Could you check a few things on this model? Use its own coordinates, in mm. A direction names the side the tool comes from. Coordinates: 2 decimals unless noted, no trailing zeros. Write each loop counter-clockwise with the first axis right and the second up, starting at its lowest first coordinate (ties: lowest second). Pieces come first, ordered by that corner, then holes.
```python
from build123d import *

# Parameters (mm, degrees)
BOSS_EXTRUDE1_DEPTH = 45.45
CUT_EXTRUDE4_DEPTH  = 1
CUT_EXTRUDE5_DEPTH  = 5
SKETCH9_R           = 1.75
CUT_EXTRUDE6_DEPTH  = 5
BOSS_EXTRUDE2_DEPTH = 5
SKETCH11_R          = 1.75
SKETCH11_R_2        = 1.715
CUT_EXTRUDE7_DEPTH  = 5
SKETCH13_R          = 3.5
CUT_EXTRUDE8_DEPTH  = 5
SKETCH13_3_R        = 11.1
CUT_EXTRUDE9_DEPTH  = 2.6
SKETCH14_W          = 50.45
SKETCH14_H          = 11.35
BOSS_EXTRUDE3_DEPTH = 5
SKETCH15_W          = 50.45
SKETCH15_H          = 11.35
BOSS_EXTRUDE4_DEPTH = 5
SKETCH17_W          = 42
SKETCH17_H          = 5
BOSS_EXTRUDE5_DEPTH = 11
BOSS_EXTRUDE6_DEPTH = 5
BOSS_EXTRUDE7_DEPTH = 5
SKETCH21_R          = 3
BOSS_EXTRUDE8_DEPTH = 15
FILLET1_R           = 5
FILLET2_R           = 5


with BuildPart() as part:
    # Sketch1 → Boss-Extrude1 (new body)
    with BuildSketch(Plane(origin=(0, 0, 0), x_dir=(1, 0, 0), z_dir=(0, 1, 0))):
        Polygon((22.725, 27.35), (22.725, 32.35), (-22.725, 32.35), (-27.725, 32.35), (-27.725, -27.35), (-27.725, -32.35), (22.725, -32.35), (22.725, -27.35), (-22.725, -27.35), (-22.725, 27.35), (0, 27.35), align=None)
    extrude(amount=BOSS_EXTRUDE1_DEPTH)

    # Sketch5 → Cut-Extrude4 (cut)
    with BuildSketch(Plane.XY.offset(-27.35)):
        with BuildLine():
            Line((0, 33.825), (22.725, 33.825))
            Line((22.725, 33.825), (22.725, 11.625))
            Line((22.725, 11.625), (0, 11.625))
            ThreePointArc((0, 11.625), (-11.1, 22.725), (0, 33.825))
        make_face()
    extrude(amount=-CUT_EXTRUDE4_DEPTH, mode=Mode.SUBTRACT)

    # Sketch6 → Cut-Extrude5 (cut)
    with BuildSketch(Plane.XY.offset(-27.35)):
        with BuildLine():
            Line((0, 26.225), (22.725, 26.225))
            Line((22.725, 26.225), (22.725, 19.225))
            Line((22.725, 19.225), (0, 19.225))
            ThreePointArc((0, 19.225), (-3.5, 22.725), (0, 26.225))
        make_face()
    extrude(amount=-CUT_EXTRUDE5_DEPTH, mode=Mode.SUBTRACT)

    # Sketch9 → Cut-Extrude6 (cut)
    with BuildSketch(Plane.XY.offset(-27.35)):
        with Locations((15.175, 37.9)):
            Circle(SKETCH9_R)
        with Locations((-15.175, 37.9)):
            Circle(SKETCH9_R)
        with Locations((15.175, 7.55)):
            Circle(SKETCH9_R)
        with Locations((-15.175, 7.55)):
            Circle(SKETCH9_R)
    extrude(amount=-CUT_EXTRUDE6_DEPTH, mode=Mode.SUBTRACT)

    # Sketch10 → Boss-Extrude2 (add)
    with BuildSketch(Plane(origin=(-22.725, 0, 0), x_dir=(0, 0, -1), z_dir=(1, 0, 0))):
        Polygon((0, 45.45), (21, 45.45), (21, 87.45), (-21, 87.45), (-21, 45.45), align=None)
    extrude(amount=-BOSS_EXTRUDE2_DEPTH)

    # Sketch11 → Cut-Extrude7 (cut)
    with BuildSketch(Plane(origin=(-22.725, 0, 0), x_dir=(0, 0, -1), z_dir=(1, 0, 0))):
        with Locations((-15.4, 81.65)):
            Circle(SKETCH11_R)
        with Locations((15.4, 81.65)):
            Circle(SKETCH11_R)
        with Locations((-15.4, 50.85)):
            Circle(SKETCH11_R_2)
        with Locations((15.4, 50.85)):
            Circle(SKETCH11_R)
    extrude(amount=-CUT_EXTRUDE7_DEPTH, mode=Mode.SUBTRACT)

    # Sketch13 → Cut-Extrude8 (cut)
    with BuildSketch(Plane(origin=(-22.725, 0, 0), x_dir=(0, 0, -1), z_dir=(1, 0, 0))):
        with Locations((0, 66.25)):
            Circle(SKETCH13_R)
    extrude(amount=-CUT_EXTRUDE8_DEPTH, mode=Mode.SUBTRACT)

    # Sketch13<3> → Cut-Extrude9 (cut)
    with BuildSketch(Plane(origin=(-22.725, 0, 0), x_dir=(0, 0, -1), z_dir=(1, 0, 0))):
        with Locations((0, 66.25)):
            Circle(SKETCH13_3_R)
    extrude(amount=-CUT_EXTRUDE9_DEPTH, mode=Mode.SUBTRACT)

    # Sketch14 → Boss-Extrude3 (add)
    with BuildSketch(Plane(origin=(0, 45.45, 0), x_dir=(1, 0, 0), z_dir=(0, 1, 0))):
        with Locations((-2.5, 26.675)):
            Rectangle(SKETCH14_W, SKETCH14_H)
    extrude(amount=BOSS_EXTRUDE3_DEPTH)

    # Sketch15 → Boss-Extrude4 (add)
    with BuildSketch(Plane(origin=(0, 45.45, 0), x_dir=(1, 0, 0), z_dir=(0, 1, 0))):
        with Locations((-2.5, -26.675)):
            Rectangle(SKETCH15_W, SKETCH15_H)
    extrude(amount=BOSS_EXTRUDE4_DEPTH)

    # Sketch17 → Boss-Extrude5 (add)
    with BuildSketch(Plane.ZY.offset(27.725)):
        with Locations((0, 89.95)):
            Rectangle(SKETCH17_W, SKETCH17_H)
    extrude(amount=-BOSS_EXTRUDE5_DEPTH)

    # Sketch19 → Boss-Extrude6 (add)
    with BuildSketch(Plane.XY.offset(21)):
        Polygon((-22.725, 50.45), (7.275, 50.45), (-16.725, 87.45), (-16.725, 92.45), (-27.725, 92.45), (-27.725, 50.45), align=None)
    extrude(amount=BOSS_EXTRUDE6_DEPTH)

    # Sketch20 → Boss-Extrude7 (add)
    with BuildSketch(Plane(origin=(0, 0, -21), x_dir=(-1, 0, 0), z_dir=(0, 0, -1))):
        Polygon((22.725, 50.45), (-7.275, 50.45), (16.725, 87.45), (16.725, 92.45), (27.725, 92.45), (27.725, 50.45), align=None)
    extrude(amount=BOSS_EXTRUDE7_DEPTH)

    # Sketch21 → Boss-Extrude8 (add)
    with BuildSketch(Plane(origin=(0, 0, 27.35), x_dir=(-1, 0, 0), z_dir=(0, 0, -1))):
        with Locations((0, 22.725)):
            Circle(SKETCH21_R)
    extrude(amount=-BOSS_EXTRUDE8_DEPTH)

    # Fillet1
    fillet1_edges = [part.edges().sort_by_distance(p)[0] for p in [
        (7.275, 50.45, 23.5),
        (7.275, 50.45, -23.5),
    ]]
    fillet(fillet1_edges, radius=FILLET1_R)

    # Fillet2
    fillet2_edges = [part.edges().sort_by_distance(p)[0] for p in [
        (-16.725, 87.45, 23.5),
        (-16.725, 87.45, -23.5),
    ]]
    fillet(fillet2_edges, radius=FILLET2_R)


solid = part.part
```
1. Please list where these lines run through material, in increasing order: line 1 along Z through (x, y) = (5, 34); line 2 along Y through (x, z) = (10.5, -27.5) (3 decimals); line 3 along Y through (x, z) = (-26.65, 0).
Verdict:
line 1: z = -32.35 to -27.35, 27.35 to 32.35
line 2: y = 0 to 11.625, 33.825 to 50.45
line 3: y = 0 to 62.75, 69.75 to 92.45
2. If we mould it in two halves opening along Z, with no side actions, what happens to faces 1 (the face through (-14.234, 9.026, -29.815)), 2 (the face through (0, 23, 27.35)), 3 (the face through (-18, 67, -26))? For each: pulls with the +Z half, pulls with the -Z half, needs draft (parallel to the pull), parting line crosses it, or undercut.
Verdict:
face 1: needs draft
face 2: undercut
face 3: pulls with the -Z half
3. On a 3-axis mill with a long thin cutter (end or side, diameter ignored), from which of +Z, -Z, +X, -X, +Y, -Y can I reach the whole of each face in a straight line? I mean faces 4 (the face through (-13.5, 38.4, -29.8)), 5 (the face through (0.65, 19.796, 37.28)), 6 (the face through (-11.097, 22.481, -27.843)). Say none if no direction works.
Verdict:
face 4: -Z
face 5: +Z
face 6: +X
4. I want a section at D-D on x = -1.5. Please give me the cut outline in (y, z), plus the area to 3 significant figures.
Verdict:
outline: (0, -32.35) - (19.56, -32.35) - (19.56, -28.35) - (11.73, -28.35) - (11.73, -27.35) - (0, -27.35) - close; (0, 27.35) - (45.45, 27.35) - (45.45, 21) - (63.98, 21) - (63.98, 26) - (50.45, 26) - (50.45, 32.35) - (25.32, 32.35) - (25.32, 42.35) - (20.13, 42.35) - (20.13, 32.35) - (0, 32.35) - close; (25.89, -32.35) - (50.45, -32.35) - (50.45, -26) - (63.98, -26) - (63.98, -21) - (45.45, -21) - (45.45, -27.35) - (33.72, -27.35) - (33.72, -28.35) - (25.89, -28.35) - close
area: 708 mm2
5. For pin 1 (11 mm diameter, centred on y = 67.5, z = 1, fed in from +X) (3 decimals); pin 2 (1 mm diameter, centred on x = -3.5, z = 30.5, fed in from +Y); pin 3 (8 mm diameter, centred on x = -8, z = 24, fed in from +Y), each with a flat end and sliding along its axis, tell me the tip position at first contact or that it passes through.
Verdict:
pin 1: stops at x = -25.325
pin 2: stops at y = 50.45
pin 3: stops at y = 80.17
6. I want a section at B-B on y = 7.55. Please give me the cut outline in (x, z) (3 decimals), plus the area to 3 significant figures.
Verdict:
outline: (-27.725, -32.35) - (-16.925, -32.35) - (-16.925, -27.35) - (-22.725, -27.35) - (-22.725, 27.35) - (22.725, 27.35) - (22.725, 32.35) - (-27.725, 32.35) - close; (-13.425, -32.35) - (13.425, -32.35) - (13.425, -27.35) - (-13.425, -27.35) - close; (16.925, -32.35) - (22.725, -32.35) - (22.725, -27.35) - (16.925, -27.35) - close
area: 743 mm2
7. I want a section at A-A on z = 0. Please give me the cut outline in (x, y) (3 decimals).
Verdict:
outline: (-27.725, 0) - (-22.725, 0) - (-22.725, 55.15) - (-25.325, 55.15) - (-25.325, 62.75) - (-27.725, 62.75) - close; (-27.725, 69.75) - (-25.325, 69.75) - (-25.325, 77.35) - (-22.725, 77.35) - (-22.725, 87.45) - (-16.725, 87.45) - (-16.725, 92.45) - (-27.725, 92.45) - close
8. I want a section at C-C on z = 15.4. Please give me the cut outline in (x, y) (3 decimals).
Verdict:
outline: (-27.725, 0) - (-22.725, 0) - (-22.725, 49.135) - (-27.725, 49.135) - close; (-27.725, 52.565) - (-22.725, 52.565) - (-22.725, 79.9) - (-27.725, 79.9) - close; (-27.725, 83.4) - (-22.725, 83.4) - (-22.725, 87.45) - (-16.725, 87.45) - (-16.725, 92.45) - (-27.725, 92.45) - close
